Geometry check sheet. Reference: the model listing, model coordinates, mm. A direction names the side the tool comes from. Coordinates: 2 decimals unless noted, no trailing zeros. Write each loop counter-clockwise with the first axis right and the second up, starting at its lowest first coordinate (ties: lowest second). Pieces come first, ordered by that corner, then holes. Notation, with made-up numbers: (13, 63.5) -> (69, 63.5) arc R22 cw to (69, 87.5) -> close; hole circle Ø8 at (69, -11.5). An arc over 180 degrees is marked (long way). Answer in a Markdown table with one row per item. Add a question column.
Q1. Section check A-A, the plane x = -113.5. Record the boundary of the cut face in (y, z), and give its area (3 significant figures).
Q2. Release check for a two-part mould opening along Y. For faces 5 (the face through (-206.065, 67.281, 0.023)), 6 (the face through (-63.92, -44.93, 0.02)), 7 (the face through (-44.84, -127.81, 0.02)) record: pulls with the +Y half, pulls with the -Y half, needs draft (parallel to the pull), parting line crosses it, or undercut.
Q3. Section check B-B, the plane x = -146.5. Record the boundary of the cut face in (y, z), and give its area (3 significant figures).
Q4. Section check C-C, the plane y = -76. Record the boundary of the cut face in (x, z), and give its area (3 significant figures).
Q5. Thickness scan on line 1 (Y direction, x = -113, z = -0.25); line 2 (Y direction, x = -95, z = -0.75); line 3 (Y direction, x = -168, z = 0.8). Record the ranges inside material, lowest first.
Q6. Section check D-D, the plane z = -0.9. Count the separate pieces of the cut face and the enclosed holes in it, and give its area (3 significant figures).
Q7. Gauge pin test, flat ends, axial feed: P1, Ø1, axis at x = -131.5, z = -0.5, coming from the -Y side; P2, Ø1.5, axis at y = -99, z = -1, coming from the +X side; P3, Ø1, axis at x = -84, z = 0, coming from the +Y side. Record the tip position at first contact, or that the pin passes through.
Q8. Tool access check on faces 1 (the face through (-26.119, -24.067, 0.023)), 2 (the face through (-224.79, 52.14, 0.02)), 3 (the face through (-205.71, -127.45, 0.02)), 4 (the face through (-98.086, -15.594, 0.023)). Record the directions out of +Z, -Z, +X, -X, +Y, -Y that give a thin tool (end or side, any length) a straight path to the whole face; none if there is none.
```python
from build123d import *

# Parameters (mm, degrees)
BOSS_EXTRUDE1_DEPTH = 2.413
SCALE1_SCALE        = 0.666666667


with BuildPart() as part:
    # Model → Boss-Extrude1 (new body, symmetric)
    with BuildSketch(Plane.XY):
        with BuildLine():
            Line((-290.681304326, -31.2683), (-258.931304326, -12.937428953))
            Line((-258.931304326, -12.937428953), (-258.931304326, -5.149171047))
            Line((-258.931304326, -5.149171047), (-290.681304326, 13.1817))
            Line((-290.681304326, 13.1817), (-290.681304326, 51.2817))
            Line((-290.681304326, 51.2817), (-258.931304326, 69.612571047))
            Line((-258.931304326, 69.612571047), (-258.931304326, 76.6817))
            Line((-258.931304326, 76.6817), (-290.681304326, 108.4317))
            Line((-290.681304326, 108.4317), (-290.681304326, 127.4817))
            ThreePointArc((-290.681304326, 127.4817), (-288.821432386, 131.971828061), (-284.331304326, 133.8317))
            Line((-284.331304326, 133.8317), (-265.281304326, 133.8317))
            Line((-265.281304326, 133.8317), (-227.181304326, 95.7317))
            Line((-227.181304326, 95.7317), (-23.981304326, 95.7317))
            Line((-23.981304326, 95.7317), (14.118695674, 133.8317))
            Line((14.118695674, 133.8317), (33.168695674, 133.8317))
            ThreePointArc((33.168695674, 133.8317), (37.658823735, 131.971828061), (39.518695674, 127.4817))
            Line((39.518695674, 127.4817), (39.518695674, 108.4317))
            Line((39.518695674, 108.4317), (7.768695674, 76.6817))
            Line((7.768695674, 76.6817), (7.768695674, 69.612571047))
            Line((7.768695674, 69.612571047), (39.518695674, 51.2817))
            Line((39.518695674, 51.2817), (39.518695674, 13.1817))
            Line((39.518695674, 13.1817), (7.768695674, -5.149171047))
            Line((7.768695674, -5.149171047), (7.768695674, -12.937428953))
            Line((7.768695674, -12.937428953), (39.518695674, -31.2683))
            Line((39.518695674, -31.2683), (39.518695674, -59.836710662))
            Line((39.518695674, -59.836710662), (10.464640386, -80.18057919))
            Line((10.464640386, -80.18057919), (7.768695674, -82.0683))
            Line((7.768695674, -82.0683), (7.768695674, -139.2183))
            Line((7.768695674, -139.2183), (39.518695674, -170.9683))
            Line((39.518695674, -170.9683), (39.518695674, -190.0183))
            ThreePointArc((39.518695674, -190.0183), (37.658823735, -194.508428061), (33.168695674, -196.3683))
            Line((33.168695674, -196.3683), (14.118695674, -196.3683))
            Line((14.118695674, -196.3683), (-23.981304326, -158.2683))
            Line((-23.981304326, -158.2683), (-227.181304326, -158.2683))
            Line((-227.181304326, -158.2683), (-265.281304326, -196.3683))
            Line((-265.281304326, -196.3683), (-284.331304326, -196.3683))
            ThreePointArc((-284.331304326, -196.3683), (-288.821432386, -194.508428061), (-290.681304326, -190.0183))
            Line((-290.681304326, -190.0183), (-290.681304326, -170.9683))
            Line((-290.681304326, -170.9683), (-258.931304326, -139.2183))
            Line((-258.931304326, -139.2183), (-258.931304326, -82.0683))
            Line((-258.931304326, -82.0683), (-290.681304326, -50.3183))
            Line((-290.681304326, -50.3183), (-290.681304326, -31.2683))
        make_face()
        Polygon((-30.331304326, -145.5683), (-68.431304326, -107.4683), (-182.731304326, -107.4683), (-220.831304326, -145.5683), align=None, mode=Mode.SUBTRACT)
        Polygon((-220.831304326, 83.0317), (-182.731304326, 44.9317), (-68.431304326, 44.9317), (-30.331304326, 83.0317), align=None, mode=Mode.SUBTRACT)
        Polygon((-201.781304326, -69.3683), (-233.531304326, -37.6183), (-233.531304326, -24.9183), (-201.781304326, 6.8317), (-182.731304326, 6.8317), (-150.981304326, -24.9183), (-150.981304326, -37.6183), (-182.731304326, -69.3683), align=None, mode=Mode.SUBTRACT)
        Polygon((-100.181304326, -37.6183), (-100.181304326, -24.9183), (-68.431304326, 6.8317), (-49.381304326, 6.8317), (-17.631304326, -24.9183), (-17.631304326, -37.6183), (-49.381304326, -69.3683), (-68.431304326, -69.3683), align=None, mode=Mode.SUBTRACT)
    extrude(amount=BOSS_EXTRUDE1_DEPTH, both=True)


with BuildPart() as part_1:
    # Scale1: scaled about (-125.200156118, -28.252377371, 0)
    add(part.part.scale(SCALE1_SCALE).moved(Location((-41.733385373, -9.417459124, 0))))


solid = part_1.part
```
Calculated:
| question | item | result |
|---|---|---|
| 1 | outline | (-114.93, -1.61) -> (-106.46, -1.61) -> (-106.46, 1.61) -> (-114.93, 1.61) -> close; (-81.06, -1.61) -> (20.54, -1.61) -> (20.54, 1.61) -> (-81.06, 1.61) -> close; (45.94, -1.61) -> (54.4, -1.61) -> (54.4, 1.61) -> (45.94, 1.61) -> close |
| 1 | area | 381 mm² |
| 2 | face 5 | pulls with the +Y half |
| 2 | face 6 | undercut |
| 2 | face 7 | pulls with the -Y half |
| 3 | outline | (-114.93, -1.61) -> (-106.46, -1.61) -> (-106.46, 1.61) -> (-114.93, 1.61) -> close; (-81.06, -1.61) -> (-38.61, -1.61) -> (-38.61, 1.61) -> (-81.06, 1.61) -> close; (-21.92, -1.61) -> (20.54, -1.61) -> (20.54, 1.61) -> (-21.92, 1.61) -> close; (45.94, -1.61) -> (54.4, -1.61) -> (54.4, 1.61) -> (45.94, 1.61) -> close |
| 3 | area | 328 mm² |
| 4 | outline | (-214.35, -1.61) -> (-36.55, -1.61) -> (-36.55, 1.61) -> (-214.35, 1.61) -> close |
| 4 | area | 572 mm² |
| 5 | line 1 | y = -114.93 to -106.46, -81.06 to 20.54, 45.94 to 54.4 |
| 5 | line 2 | y = -114.93 to -106.46, -81.06 to -48.02, -12.51 to 20.54, 45.94 to 54.4 |
| 5 | line 3 | y = -114.93 to -106.46, -85.51 to -55.66, -4.86 to 24.98, 45.94 to 54.4 |
| 6 | separate pieces | 1 |
| 6 | enclosed holes | 4 |
| 6 | area | 27,200 mm² |
| 7 | P1 | stops at y = -114.93 |
| 7 | P2 | stops at x = -36.55 |
| 7 | P3 | stops at y = 54.4 |
| 8 | face 1 | +Z, -Z, +X |
| 8 | face 2 | +Z, -Z, -X |
| 8 | face 3 | +Z, -Z, -Y |
| 8 | face 4 | +Z, -Z |
